Source: CAD feature listing. Evaluate the final solid. Frame: model axes, mm. A direction names the side the tool comes from. Give positions to 0.01 mm unless a question says otherwise; leave off trailing zeros. Write each loop counter-clockwise with the first axis right and the second up, starting at its lowest first coordinate (ties: lowest second). Pieces come first, ordered by that corner, then holes. Notation, with made-up numbers: (53.5, 22.5) -> (94.5, 22.5) arc R35 ccw to (94.5, 57.5) -> close; hole circle Ø9 at (22.25, -26.75). An arc over 180 degrees is marked (long way). Use one line per item in the form item = value. Start each with the question number.
(1) Cut plane C-C, the plane y = 2. Output: boundary loops of the cut face in (x, z).
(2) Draft query along Y for faces 6 (the face through (9.322, 10.607, -21.245)), 7 (the face through (0, 0, 18)), 8 (the face through (13, 10.1, 18)). Return one class per face: pulls with the +Y half, pulls with the -Y half, needs draft (parallel to the pull), parting line crosses it, or undercut.
(3) Cut plane A-A, the plane x = 0. Output: boundary loops of the cut face in (y, z), and give its area (3 significant figures).
(4) Cut plane B-B, the plane y = 5.25. Output: boundary loops of the cut face in (x, z).
(5) Set-up query: faces 1 (the face through (13.738, 10.607, 18.695)), 2 (the face through (8, 11.1, 19)), 3 (the face through (8.9, 10.1, -20.5)), 4 (the face through (20, 4, -10)), 5 (the face through (-23.06, 10.61, 2.55)). Return all of +Z, -Z, +X, -X, +Y, -Y with unobstructed straight access to the full face (end or side cutting, diameter ignored); none if empty.
(6) First-contact query: P1, Ø4, axis at x = 19.5, y = 8.5, coming from the +Z side; P2, Ø4, axis at y = 7.5, z = -5, coming from the +X side; P3, Ø1, axis at x = 21.5, y = 1, coming from the +Z side. Flat tips, straight axial feed; report the tip coordinate or a pass-through.
(7) Material intervals for line 1 along Y through (x, z) = (6.5, -22); line 2 along X through (y, z) = (8.5, 7); line 3 along Z through (x, y) = (13, 8.5), sorted ascending. Write a range as from..to.
from build123d import *
from build123d.topology import SkipClean

# Parameters (mm, degrees)
SKETCH1_W          = 2
SKETCH1_H          = 11.1
SKETCH1_W_2        = 5
SKETCH1_H_2        = 4
SKETCH1_W_3        = 1.2
SKETCH1_H_3        = 1
CUT_EXTRUDE1_DEPTH = 1


with BuildPart() as part:
    # Sketch1 → Revolve1 (revolve)
    with BuildSketch(Plane.XY, mode=Mode.PRIVATE) as revolve1_sk:
        with Locations((21, 5.55)):
            Rectangle(SKETCH1_W, SKETCH1_H)
        with Locations((24.5, 2)):
            Rectangle(SKETCH1_W_2, SKETCH1_H_2)
        with Locations((22.6, 10.6)):
            Rectangle(SKETCH1_W_3, SKETCH1_H_3)
        Polygon((17, 0), (20, 11.1), (20, 0), align=None)
    revolve(revolve1_sk.sketch.rotate(Axis((0, 0, 0), (0, 1, 0)), 90), axis=Axis((0, 0, 0), (0, 1, 0)))  # turned: the seam where the file's is

    # Sketch3 → Cut-Extrude1 (cut)
    with SkipClean():  # keep this step's faces unmerged: merging them makes the solid invalid here
        with BuildSketch(Plane(origin=(0, 11.1, 0), x_dir=(1, 0, 0), z_dir=(0, 1, 0))):
            with BuildLine():
                ThreePointArc((23.2, 0), (21.721311586, 8.150130242), (17.473739399, 15.261337799))
                Line((17.473739399, 15.261337799), (16.569925293, 14.471958257))
                ThreePointArc((16.569925293, 14.471958257), (20.59779547, 7.728571782), (22, 0))
                ThreePointArc((22, 0), (21.355762595, -5.285016934), (19.460781455, -10.260506087))
                Line((19.460781455, -10.260506087), (20.522278625, -10.820170056))
                ThreePointArc((20.522278625, -10.820170056), (22.520622373, -5.573290585), (23.2, 0))
            make_face()
            with BuildLine():
                Line((-18.616249655, -11.723278074), (-19.631681454, -12.362729605))
                ThreePointArc((-19.631681454, -12.362729605), (-9.18901176, -21.302630421), (4.47983653, -22.763371118))
                Line((4.47983653, -22.763371118), (4.248120847, -21.585955371))
                ThreePointArc((4.248120847, -21.585955371), (-8.713718048, -20.200770227), (-18.616249655, -11.723278074))
            make_face()
            with BuildLine():
                Line((-0.8445318, 21.983784161), (-0.890597171, 23.182899661))
                ThreePointArc((-0.890597171, 23.182899661), (-13.854113232, 18.609232831), (-21.953575929, 7.50203332))
                Line((-21.953575929, 7.50203332), (-20.81804614, 7.113997113))
                ThreePointArc((-20.81804614, 7.113997113), (-13.137521169, 17.646686305), (-0.8445318, 21.983784161))
            make_face()
        extrude(amount=-CUT_EXTRUDE1_DEPTH, mode=Mode.SUBTRACT)


solid = part.part
Geometry says:
q1.outline = circle Ø54 at (0, 0); hole circle Ø35.08 at (0, 0)
q2.face_6 = needs draft
q2.face_7 = pulls with the -Y half
q2.face_8 = undercut
q3.outline = (0, -27) -> (4, -27) -> (4, -22) -> (10.1, -22) -> (10.1, -23.2) -> (11.1, -23.2) -> (11.1, -20) -> (0, -17) -> close; (0, 17) -> (11.1, 20) -> (11.1, 22) -> (4, 22) -> (4, 27) -> (0, 27) -> close
q3.area = 119 mm^2
q4.outline = circle Ø44 at (0, 0); hole circle Ø36.84 at (0, 0)
q5.face_1 = +Z, +X, +Y
q5.face_2 = +Z, -Z, +X, -X, +Y
q5.face_3 = -Z, +X
q5.face_4 = none
q5.face_5 = -X, +Y
q6.P1 = 14.26
q6.P2 = 21.79
q6.P3 = 16.97
q7.line_1 = 0..4, 10.1..11.1
q7.line_2 = -20.86..-17.98, 17.98..20.86
q7.line_3 = -17.75..-14.26, 14.26..17.75
